The drawing under review shows one solid part. Ordinate dimensions are in mm from its lowest x, y, z. Round coordinates to 2 decimals unless told otherwise and drop trailing zeros. Write each loop counter-clockwise with the first axis right and the second up, starting at its lowest first coordinate (ties: lowest second). Pieces come first, ordered by that corner, then holes.
Item 1: To check wall thickness, follow L1, parallel to X at y = 59.5, z = 11.25; L2, parallel to Y at x = 16.7, z = 11.1; L3, parallel to X at y = 53, z = 1.25. State the ranges of each line that lie inside material, in increasing order.
Item 2: Draft analysis for pull direction X (two halves, no side actions). For the marked faces 1, 2, 3 and 4, state which applies: +X half, -X half, draft (parallel to the pull), parting line (faces both ways), or undercut.
Item 3: Add section A-A (x = 32). Give the boundary of the cut face in (y, z), plus the area to 3 significant figures.
Item 4: Add section D-D (x = 23). Give the boundary of the cut face in (y, z), plus the area to 3 significant figures.
Item 5: Clearance check with flat-ended pins moving along their axes: pin 1 Ø3.5 at (y, z) = (7, 5.207) entering from -X; pin 2 Ø2.5 at (y, z) = (35, 5.207) entering from +X. State where each tip first meets the part, or that it passes through.
Item 6: Add section C-C (z = 8). Give the boundary of the cut face in (x, y), plus the area to 3 significant figures.
Item 7: Add section B-B (y = 55.25). Give the boundary of the cut face in (x, z), plus the area to 3 significant figures.
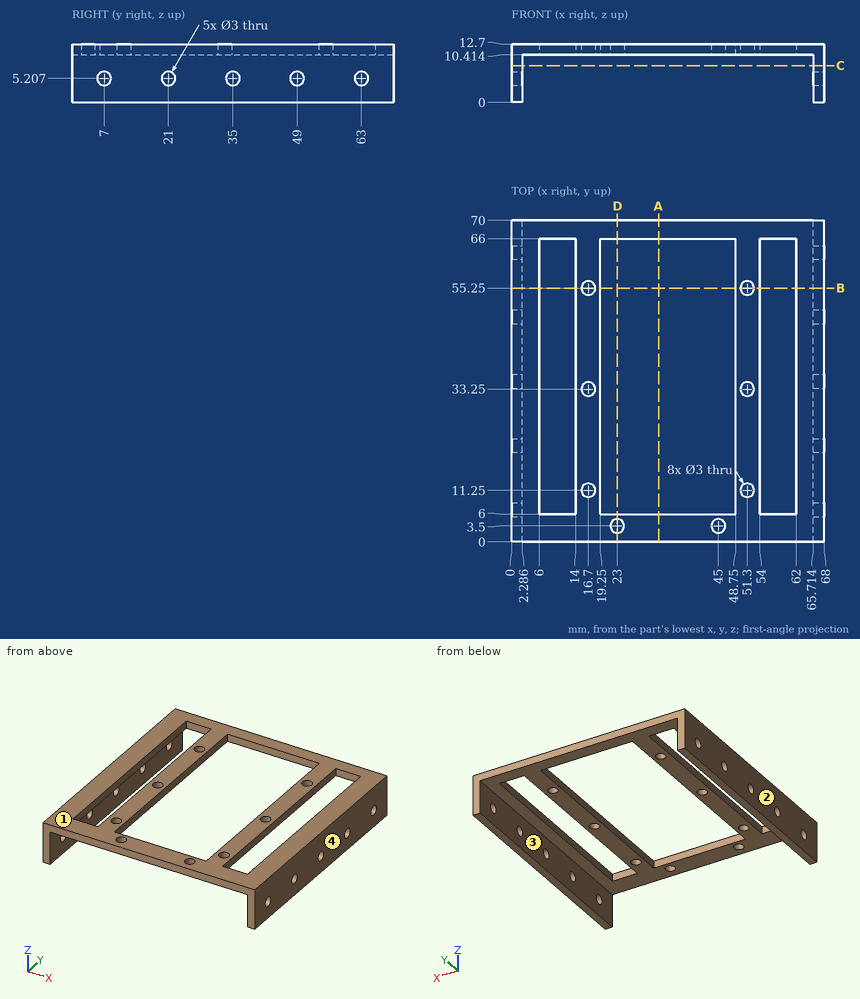
Numbers:
1. L1: x = 0 to 6, 14 to 19.25, 48.75 to 54, 62 to 68
1. L2: y = 0 to 9.75, 12.75 to 31.75, 34.75 to 53.75, 56.75 to 70
1. L3: x = 0 to 2.29, 65.71 to 68
2. face 1: draft
2. face 2: -X half
2. face 3: undercut
2. face 4: +X half
3. outline: (0, 10.41) - (6, 10.41) - (6, 12.7) - (0, 12.7) - close; (66, 10.41) - (70, 10.41) - (70, 12.7) - (66, 12.7) - close
3. area: 22.9 mm2
4. outline: (0, 10.41) - (2, 10.41) - (2, 12.7) - (0, 12.7) - close; (5, 10.41) - (6, 10.41) - (6, 12.7) - (5, 12.7) - close; (66, 10.41) - (70, 10.41) - (70, 12.7) - (66, 12.7) - close
4. area: 16.0 mm2
5. pin 1: stops at x = 0
5. pin 2: passes through
6. outline: (0, 0) - (2.29, 0) - (2.29, 70) - (0, 70) - close; (65.71, 0) - (68, 0) - (68, 70) - (65.71, 70) - close
6. area: 320 mm2
7. outline: (0, 0) - (2.29, 0) - (2.29, 10.41) - (6, 10.41) - (6, 12.7) - (0, 12.7) - close; (14, 10.41) - (15.2, 10.41) - (15.2, 12.7) - (14, 12.7) - close; (18.2, 10.41) - (19.25, 10.41) - (19.25, 12.7) - (18.2, 12.7) - close; (48.75, 10.41) - (49.8, 10.41) - (49.8, 12.7) - (48.75, 12.7) - close; (52.8, 10.41) - (54, 10.41) - (54, 12.7) - (52.8, 12.7) - close; (62, 10.41) - (65.71, 10.41) - (65.71, 0) - (68, 0) - (68, 12.7) - (62, 12.7) - close
7. area: 85.3 mm2
